Job drawing, mm, ordinate dimensions from the low corner. One solid piece. A direction names the side the tool comes from. Give positions to 0.01 mm unless a question says otherwise; leave off trailing zeros. Order: outer loops, then holes, each group sorted by start corner. A loop starts at its lowest first (then second) coordinate and runs counter-clockwise, first axis right, second up.
Item 1: Band-saw the part on B-B on z = 3.75. Give the cut face in (x, y), plus the area to 3 significant figures.
Item 2: Which spindle directions (+Z, -Z, +X, -X, +Y, -Y) get a long thin tool onto all of the face, cutting with end or side? Do the marked faces 5, 6 and 7. Say none if no direction does.
Item 3: Two-plate mould, pull along X, no slides. Class the marked faces 1, 2, 3 and 4: released by +X, released by -X, zero draft, split by the parting line, or undercut.
Item 4: Band-saw the part on A-A on x = 3. Give the cut face in (y, z), plus the area to 3 significant figures.
Item 5: Flat gauge pins, fed straight in: P1, Ø4, axis at x = 31, z = 4.5, coming from the -Y side; P2, Ø2, axis at y = 20, z = 5, coming from the +X side; P3, Ø2, axis at x = 26.5, z = 5, coming from the +Y side; P4, Ø4, axis at x = 3, z = 8.5, coming from the -Y side. Where does each tip first touch, or does it go through?
Item 6: Band-saw the part on C-C on x = 22.5. Give the cut face in (y, z), plus the area to 3 significant figures.
Item 7: Wall check: L1, parallel to X at y = 5.5, z = 10; L2, parallel to Y at x = 27, z = 11.25; L3, parallel to Z at x = 11, y = 23.75. Give the ranges that are in metal, low to high.
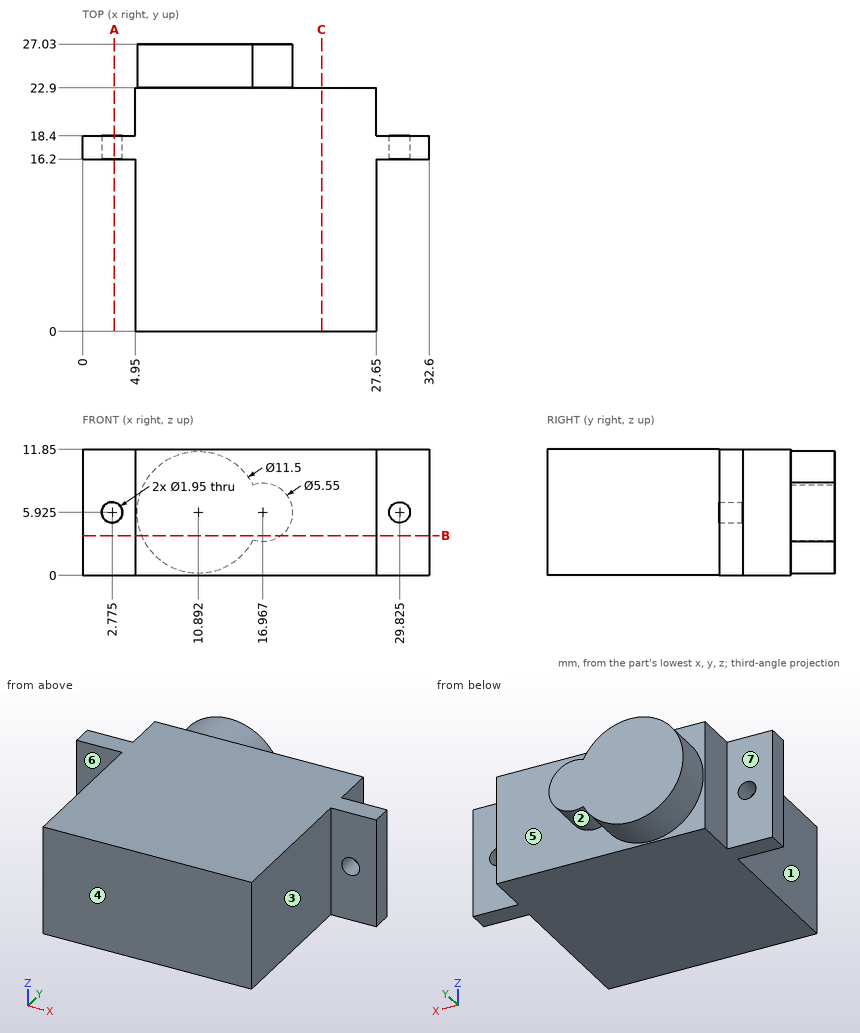
The answers:
1. outline: (0, 16.2) - (4.95, 16.2) - (4.95, 0) - (27.65, 0) - (27.65, 16.2) - (32.6, 16.2) - (32.6, 18.4) - (27.65, 18.4) - (27.65, 22.9) - (18.69, 22.9) - (18.69, 27.03) - (5.57, 27.03) - (5.57, 22.9) - (4.95, 22.9) - (4.95, 18.4) - (0, 18.4) - close
1. area: 596 mm2
2. face 5: +Y
2. face 6: +Z, -Z, -X, -Y
2. face 7: +Z, -Z, -X, +Y
3. face 1: released by -X
3. face 2: undercut
3. face 3: released by +X
3. face 4: zero draft
4. outline: (16.2, 0) - (18.4, 0) - (18.4, 4.98) - (16.2, 4.98) - close; (16.2, 6.87) - (18.4, 6.87) - (18.4, 11.85) - (16.2, 11.85) - close
4. area: 21.9 mm2
5. P1: stops at y = 16.2
5. P2: stops at x = 27.65
5. P3: stops at y = 22.9
5. P4: stops at y = 0
6. outline: (0, 0) - (22.9, 0) - (22.9, 11.85) - (0, 11.85) - close
6. area: 271 mm2
7. L1: x = 4.95 to 27.65
7. L2: y = 0 to 22.9
7. L3: z = 0.18 to 11.67
